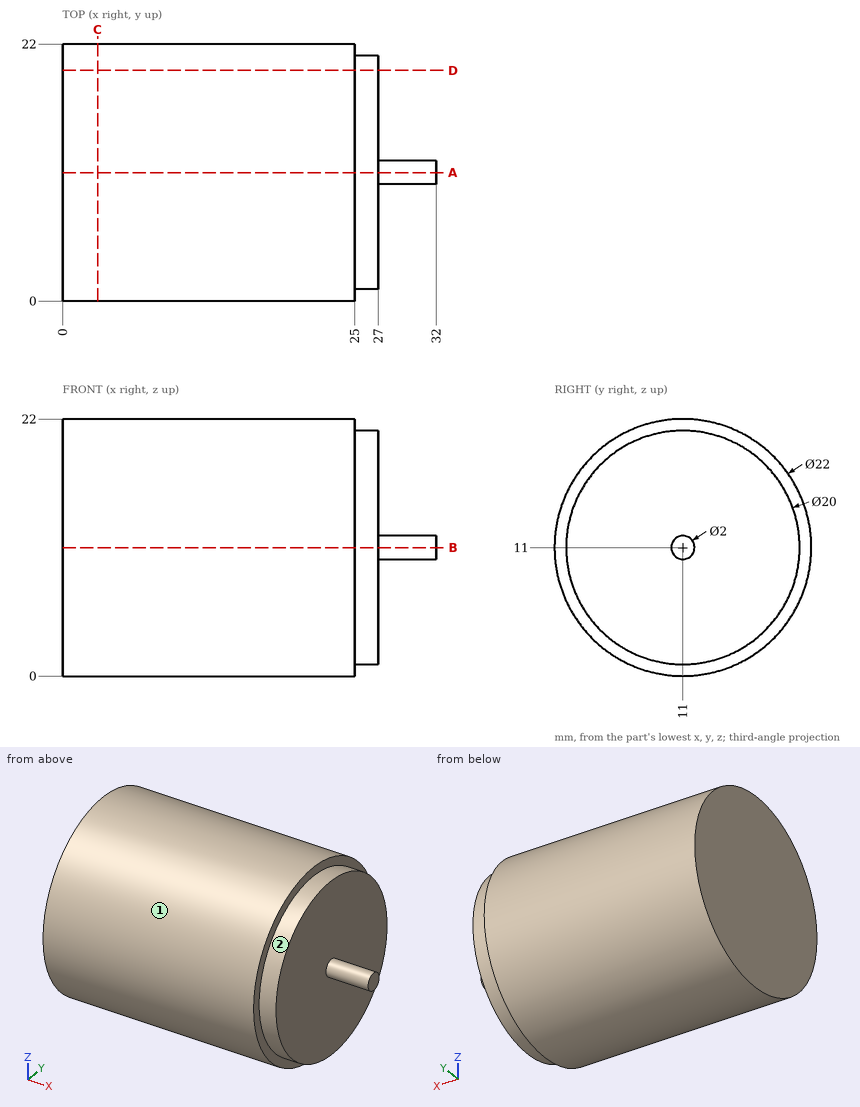
Can you work these out from the drawing? Everything is in mm from the part's minimum corner. A direction names the side the tool comes from. Give positions to 0.01 mm unless a question says otherwise; leave off trailing zeros. Write each loop counter-clockwise with the first axis right and the second up, starting at its lowest first coordinate (ties: lowest second). Pieces come first, ordered by that corner, then holes. Notation, with made-up numbers: M 50.5,50 L 66.5,50 A20 cw 66.5,74 Z; hole C -27.5,-8 d11. An arc over 180 degrees is marked long. Answer in a Markdown table with one row per item. Add a question column.
Item 1: For pin 1 Ø1.5 at (y, z) = (12.5, 11) entering from +X; pin 2 Ø2 at (x, y) = (13, 13.5) entering from -Z; pin 3 Ø3 at (x, y) = (11.5, 18.5) entering from +Z; pin 4 Ø4 at (x, y) = (26.5, 18) entering from +Z, each with a flat end and sliding along its axis, tell me the tip position at first contact or that it passes through.
Item 2: Imagine slicing it at A-A, the plane y = 11. Write out the boundary of the cut face in (x, z), plus the area to 3 significant figures.
Item 3: Imagine slicing it at C-C, the plane x = 3. Write out the boundary of the cut face in (y, z).
Item 4: Please list where these lines run through material, in increasing order: L1, parallel to X at y = 3.5, z = 7.75; L2, parallel to X at y = 2.5, z = 16.5; L3, parallel to Y at x = 7.5, z = 10.
Item 5: Imagine slicing it at D-D, the plane y = 19.75. Write out the boundary of the cut face in (x, z).
Item 6: On a 3-axis mill with a long thin cutter (end or side, diameter ignored), from which of +Z, -Z, +X, -X, +Y, -Y can I reach the whole of each face in a straight line? I mean the marked faces 1 and 2. Say none if no direction works.
Evaluation:
| question | item | result |
|---|---|---|
| 1 | pin 1 | stops at x = 32 |
| 1 | pin 2 | stops at z = 0.1 |
| 1 | pin 3 | stops at z = 20.22 |
| 1 | pin 4 | stops at z = 20.42 |
| 2 | outline | M 0,0 L 25,0 L 25,1 L 27,1 L 27,10 L 32,10 L 32,12 L 27,12 L 27,21 L 25,21 L 25,22 L 0,22 Z |
| 2 | area | 600 mm² |
| 3 | outline | C 11,11 d22 |
| 4 | L1 | x = 0 to 27 |
| 4 | L2 | x = 0 to 25 |
| 4 | L3 | y = 0.05 to 21.95 |
| 5 | outline | M 0,4.33 L 25,4.33 L 25,6.16 L 27,6.16 L 27,15.84 L 25,15.84 L 25,17.67 L 0,17.67 Z |
| 6 | face 1 | +X, -X |
| 6 | face 2 | +X |
